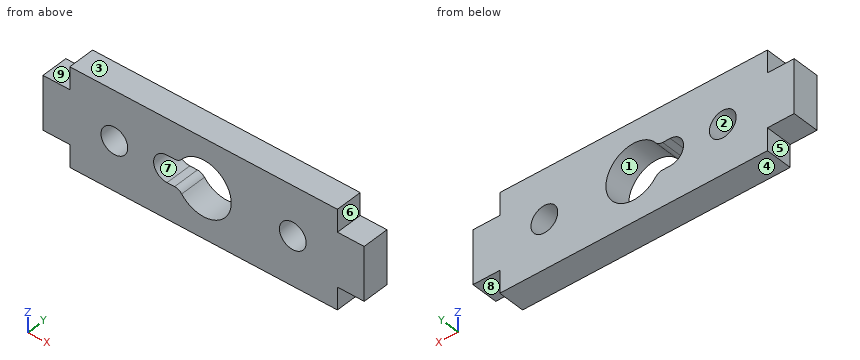
Autodesk Inventor part; units mm, degrees
ref_plane "YZ Plane" through (0, 0, 0) normal (1, 0, 0) x (0, 1, 0)
ref_plane "XZ Plane" through (0, 0, 0) normal (0, 1, 0) x (-1, 0, 0)
ref_plane "XY Plane" through (0, 0, 0) normal (0, 0, 1) x (1, 0, 0)
sketch "Sketch1" plane through (0, 0, 0) normal (0, 1, 0) x (-1, 0, 0)
  line L0 (0, 0) -> (0, -3)
  line L1 (0, -3) -> (3, -3)
  line L2 (3, -3) -> (3, -5.5)
  line L3 (3, -5.5) -> (33, -5.5)
  line L4 (33, -5.5) -> (33, -3)
  line L5 (33, -3) -> (36, -3)
  line L6 (36, -3) -> (36, 3)
  line L7 (36, 3) -> (33, 3)
  line L8 (33, 3) -> (33, 5.5)
  line L9 (33, 5.5) -> (3, 5.5)
  line L10 (3, 5.5) -> (3, 3)
  line L11 (3, 3) -> (0, 3)
  line L12 (0, 3) -> (0, 0)
  circle A0 centre (28, 0) radius 1.5
  line L13 (0, 0) -> (8, 0)
  circle A1 centre (8, 0) radius 1.5
  line L14 (22.1, 1.5) -> (21.2496, 1.5)
  line L15 (22.1, -1.5) -> (21.2496, -1.5)
  arc A2 (22.1, -1.5) -> (22.1, 1.5) centre (22.1, 0) ccw
  arc A3 (20.457, 1.8902) -> (20.457, -1.8902) centre (18, 0) ccw
  arc A4 (20.457, 1.8902) -> (21.2496, 1.5) centre (21.2496, 2.5) ccw
  arc A5 (21.2496, -1.5) -> (20.457, -1.8902) centre (21.2496, -2.5) ccw
  point P0 (20.7129, 1.5)
  point P1 (20.7129, -1.5)
  dimension "d15" = 3
  dimension "d16" = 3
  dimension "d17" = 2.5
  dimension "d18" = 30
  dimension "d19" = 3
  dimension "d20" = 6
  dimension "d21" = 2.5
  dimension "d22" = 30
  dimension "d25" = 3
  dimension "d26" = 8
  dimension "d27" = 3
  dimension "d30" = 1
  dimension "d31" = 8
  dimension "d32" = 11
  dimension "d33" = 20
extrude "Extrusion1" add sketch "Sketch1" along normal blind 3
properties part number "Laser Mount Plate" material "Polycarbonate, Smoke"
Model file for the job. Use its own axes, mm. Face numbers are marked on the shaded views. A direction names the side the tool comes from. Give positions to 0.01 mm unless a question says otherwise; leave off trailing zeros. Loops run counter-clockwise (first coordinate to the right, second up) from the corner with the lowest first, then second, coordinate; pieces in that order, holes last. Notation, with made-up numbers: M 86.25,22.25 L 123.25,22.25 A8 cw 123.25,36.25 Z; hole C 50,36 d1. An arc over 180 degrees is marked long. Use one line per item in the form item = value.
Item 1: Slice it at B-B on x = -28. List the corners of the cut face in (y, z), and give its area (3 significant figures).
Filled in:
outline = M 0,-5.5 L 3,-5.5 L 3,-1.5 L 0,-1.5 Z; M 0,1.5 L 3,1.5 L 3,5.5 L 0,5.5 Z
area = 24.0 mm^2
Item 2: Slice it at D-D on x = -18. List the corners of the cut face in (y, z).
Filled in:
outline = M 0,-5.5 L 3,-5.5 L 3,-3.1 L 0,-3.1 Z; M 0,3.1 L 3,3.1 L 3,5.5 L 0,5.5 Z
Item 3: Two-plate mould, pull along Z, no slides. Class the marked faces 1, 2, 3 and 4: released by +Z, released by -Z, zero draft, split by the parting line, or undercut.
Filled in:
face_1 = undercut
face_2 = undercut
face_3 = released by +Z
face_4 = released by -Z
Item 4: Flat gauge pins, fed straight in: pin 1 Ø1.5 at (x, y) = (-1, 1.5) entering from -Z; pin 2 Ø1.5 at (x, y) = (-34, 1) entering from +Z; pin 3 Ø1.5 at (y, z) = (1, 1.5) entering from +X; pin 4 Ø0.8 at (y, z) = (1, -4.5) entering from -X. Where does each tip first touch, or does it go through?
Filled in:
pin_1 = -3
pin_2 = 3
pin_3 = 0
pin_4 = -33
Item 5: Slice it at C-C on y = 2.2. List the corners of the cut face in (x, z).
Filled in:
outline = M -36,-3 L -33,-3 L -33,-5.5 L -3,-5.5 L -3,-3 L 0,-3 L 0,3 L -3,3 L -3,5.5 L -33,5.5 L -33,3 L -36,3 Z; hole C -28,0 d3; hole M -22.1,-1.5 L -21.25,-1.5 A1 cw -20.46,-1.89 A3.1 ccw long -20.46,1.89 A1 cw -21.25,1.5 L -22.1,1.5 A1.5 ccw Z; hole C -8,0 d3
Item 6: Which spindle directions (+Z, -Z, +X, -X, +Y, -Y) get a long thin tool onto all of the face, cutting with end or side? Do the marked faces 5, 6, 7, 8 and 9. Say none if no direction does.
Filled in:
face_5 = -Z, -X, +Y, -Y
face_6 = +Z, +X, +Y, -Y
face_7 = +Y, -Y
face_8 = -Z, +X, +Y, -Y
face_9 = +Z, -X, +Y, -Y
Item 7: Slice it at A-A on z = 0. List the corners of the cut face in (x, y), and give its area (3 significant figures).
Filled in:
outline = M -36,0 L -29.5,0 L -29.5,3 L -36,3 Z; M -26.5,0 L -23.6,0 L -23.6,3 L -26.5,3 Z; M -14.9,0 L -9.5,0 L -9.5,3 L -14.9,3 Z; M -6.5,0 L 0,0 L 0,3 L -6.5,3 Z
area = 63.9 mm^2
Item 8: Drill centre lines: L1, parallel to Z at x = -22, y = 2.5; L2, parallel to Z at x = -18, y = 1.3; L3, parallel to X at y = 2.65, z = -1. Where is each one in solid material? Low to high.
Filled in:
L1 = -5.5 to -1.5, 1.5 to 5.5
L2 = -5.5 to -3.1, 3.1 to 5.5
L3 = -36 to -29.12, -26.88 to -23.22, -15.07 to -9.12, -6.88 to 0
